CAD build for the part. Positions are in the model's coordinates, mm. A direction names the side the tool comes from. Give positions to 0.01 mm unless a question says otherwise; leave off trailing zeros. Order: outer loops, then holes, each group sorted by start corner. A loop starts at its lowest first (then second) coordinate and runs counter-clockwise, first axis right, second up.
Autodesk Inventor part; units mm, degrees
ref_plane "YZ Plane" through (0, 0, 0) normal (1, 0, 0) x (0, 1, 0)
ref_plane "XZ Plane" through (0, 0, 0) normal (0, 1, 0) x (-1, 0, 0)
ref_plane "XY Plane" through (0, 0, 0) normal (0, 0, 1) x (1, 0, 0)
sketch "草圖1" plane through (0, 0, 0) normal (0, 0, 1) x (1, 0, 0)
  line L0 (50, 0) -> (50, 100)
  line L1 (50, 100) -> (0, 100)
  line L2 (0, 100) -> (0, 0)
  line L3 (50, 0) -> (33, 0)
  line L4 (33, 0) -> (24.5, 0)
  circle A0 centre (17, 3) radius 1.5
  circle A1 centre (35, 3) radius 1.5
  line L5 (0, 0) -> (50, 0)
  dimension "d0" = 50
  dimension "d4" = 3
  dimension "d5" = 100
  dimension "d7" = 3
  dimension "d22" = 18
  dimension "d23" = 3
  dimension "d24" = 15
extrude "擠出1" add sketch "草圖1" along normal blind 20
sketch "草圖2" plane through (0, 0, 0) normal (0, -1, 0) x (1, 0, 0)
  line L0 (0, 20) -> (50, 20)
  line L1 (0, 0) -> (50, 0)
  line L2 (0, 0) -> (0, 20)
  line L3 (50, 0) -> (50, 20)
  line L4 (50, 5) -> (0, 5)
  line L5 (0, 5) -> (0, 15)
  line L6 (0, 15) -> (50, 15)
  line L7 (50, 15) -> (50, 5)
  point P0 (15, 22.5)
  point P1 (0, 5)
  dimension "d13" = 0
  dimension "d14" = 0
  dimension "d15" = 5
  dimension "d16" = 10
extrude "擠出2" cut sketch "草圖2" against normal blind 20 contours L6 L3 L4 L2
sketch "草圖3" plane through (0, 0, 0) normal (0, 0, -1) x (-1, 0, 0)
  circle A0 centre (-25, 80) radius 10
  line L0 (-50, 100) -> (0, 100)
  line L1 (0, 100) -> (0, 0)
  circle A1 centre (-8.821, 80) radius 2.067
  circle A2 centre (-41.179, 80) radius 2.067
  line L2 (-25, 80) -> (-8.821, 80)
  line L3 (-25, 80) -> (-41.179, 80)
  dimension "d17" = 20
  dimension "d18" = 20
  dimension "d19" = 25
  dimension "d27" = 4.134
  dimension "d29" = 4.134
  dimension "d30" = 16.179
  dimension "d31" = 16.179
  dimension "d32" = 0
  dimension "d33" = 0
  dimension "d34" = 0
  dimension "d35" = 0
extrude "擠出3" cut sketch "草圖3" against normal blind 20
properties part number "汽缸"
1. 3-axis set-ups, long thin cutter, end or side, ignore diameter. For faces 4 (the cylindrical face through (19.62, 88.43, 9.86)), 5 (the flat face through (25, 20, 10)): which of +Z, -Z, +X, -X, +Y, -Y reach the whole face in a straight line?
2. Mould opens along X. For faces 1 (the flat face through (0, 51, 10)), 2 (the flat face through (25, 10, 5)), 3 (the cylindrical face through (9.269, 77.982, 9.86)) say: released by +X, released by -X, zero draft, split by the parting line, or undercut.
3. Saw through at B-B on x = 25. Give the cut face in (y, z), plus the area to 3 significant figures.
4. Saw through at D-D on y = 3. Give the cut face in (x, z).
5. Saw through at C-C on z = 11.5. Give the cut face in (x, y).
6. Wall check: line 1 (X direction, y = 3, z = 3.8); line 2 (Y direction, x = 25, z = 12); line 3 (Y direction, x = 17, z = 16.9). Give the ranges that are in metal, low to high.
7. Saw through at A-A on x = 17. Give the cut face in (y, z), plus the area to 3 significant figures.
8. Pin check, flat tips, straight feed: P1, Ø6, axis at x = 39, y = 42, coming from the -Z side; P2, Ø12, axis at x = 25, y = 80, coming from the +Z side. Stop position of each tip, or through.
Reported:
1. face 4: +Z, -Z
1. face 5: +X, -X, -Y
2. face 1: released by -X
2. face 2: zero draft
2. face 3: undercut
3. outline: (0, 0) - (70, 0) - (70, 20) - (0, 20) - (0, 15) - (20, 15) - (20, 5) - (0, 5) - close; (90, 0) - (100, 0) - (100, 20) - (90, 20) - close
3. area: 1,400 mm2
4. outline: (0, 0) - (15.5, 0) - (15.5, 5) - (0, 5) - close; (0, 15) - (15.5, 15) - (15.5, 20) - (0, 20) - close; (18.5, 0) - (33.5, 0) - (33.5, 5) - (18.5, 5) - close; (18.5, 15) - (33.5, 15) - (33.5, 20) - (18.5, 20) - close; (36.5, 0) - (50, 0) - (50, 5) - (36.5, 5) - close; (36.5, 15) - (50, 15) - (50, 20) - (36.5, 20) - close
5. outline: (0, 20) - (50, 20) - (50, 100) - (0, 100) - close; hole circle Ø4.13 at (8.82, 80); hole circle Ø20 at (25, 80); hole circle Ø4.13 at (41.18, 80)
6. line 1: x = 0 to 15.5, 18.5 to 33.5, 36.5 to 50
6. line 2: y = 20 to 70, 90 to 100
6. line 3: y = 0 to 1.5, 4.5 to 74, 86 to 100
7. outline: (0, 0) - (1.5, 0) - (1.5, 5) - (0, 5) - close; (0, 15) - (1.5, 15) - (1.5, 20) - (0, 20) - close; (4.5, 0) - (74, 0) - (74, 20) - (4.5, 20) - (4.5, 15) - (20, 15) - (20, 5) - (4.5, 5) - close; (86, 0) - (100, 0) - (100, 20) - (86, 20) - close
7. area: 1,530 mm2
8. P1: stops at z = 0
8. P2: passes through
